Part model, mm, in its own coordinate system. Face numbers are marked on the shaded views. A direction names the side the tool comes from. Round coordinates to 2 decimals unless told otherwise and drop trailing zeros. Loops run counter-clockwise (first coordinate to the right, second up) from the corner with the lowest first, then second, coordinate; pieces in that order, holes last. Notation, with made-up numbers: (6.25, 82.25) -> (54.25, 82.25) arc R13 ccw to (54.25, 97.25) -> close; hole circle Ø1 at (-10, -27). An arc over 180 degrees is marked (long way). Answer as CSV lines item,"result".
Autodesk Inventor part; units mm, degrees
ref_plane "YZ Plane" through (0, 0, 0) normal (1, 0, 0) x (0, 1, 0)
ref_plane "XZ Plane" through (0, 0, 0) normal (0, 1, 0) x (-1, 0, 0)
ref_plane "XY Plane" through (0, 0, 0) normal (0, 0, 1) x (1, 0, 0)
sketch "Sketch1" plane through (0, 0, 0) normal (1, 0, 0) x (0, 1, 0)
  line L0 (12.954, 12.7) -> (12.954, -12.954)
  line L1 (12.954, -12.954) -> (-12.954, -12.954)
  line L2 (-12.954, -12.954) -> (-12.954, 12.7)
  line L3 (12.954, 17.78) -> (18.034, 17.78)
  line L4 (18.034, 17.78) -> (18.034, -18.034)
  line L5 (18.034, -18.034) -> (-18.034, -18.034)
  line L6 (-18.034, -18.034) -> (-18.034, 17.78)
  line L7 (-18.034, 17.78) -> (-12.954, 17.78)
  line L8 (12.954, 12.7) -> (12.954, 17.78)
  line L9 (-12.954, 12.7) -> (-12.954, 17.78)
  point P0 (0, 0)
extrude "Extrusion1" add sketch "Sketch1" along normal blind 76.2
sketch "Sketch3" plane through (76.2, 18.034, 17.78) normal (0, 1, 0) x (1, 0, 0)
  circle A0 centre (-12.7, 18.034) radius 2.4892
  line L0 (-76.2, 35.814) -> (0, 35.814)
  line L1 (0, 0) -> (0, 30.734)
  circle A1 centre (-25.4, 18.034) radius 2.4892
  circle A2 centre (-38.1, 18.034) radius 2.4892
  circle A3 centre (-50.8, 18.034) radius 2.4892
  circle A4 centre (-63.5, 18.034) radius 2.4892
  point P0 (-76.2, 17.78)
  point P1 (-63.5, 35.814)
  dimension "d11" = 4.9784
  dimension "d13" = 12.7
  dimension "d14" = 12.7
  dimension "d17" = 12.7
  dimension "d36" = 4.9784
  dimension "d37" = 12.7
extrude "Extrusion6" cut sketch "Sketch3" against normal blind 66.675
sketch "Sketch6" plane through (0, 0, 0) normal (-1, 0, 0) x (0, 0, 1)
  line L0 (-18.034, 18.034) -> (17.78, 18.034)
  line L1 (-18.034, 18.034) -> (-49.784, 18.034)
  line L2 (17.78, -18.034) -> (-18.034, -18.034)
  line L3 (-49.784, 18.034) -> (-18.034, -18.034)
  line L4 (-18.034, -18.034) -> (-18.034, 18.034)
  point P0 (0, 0)
  dimension "d40" = 31.75
extrude "Extrusion7" add sketch "Sketch6" against normal blind 25.4
sketch "Sketch7" plane through (0, 18.034, 17.78) normal (0, 1, 0) x (1, 0, 0)
  circle A0 centre (38.1, 18.034) radius 2.4892
  circle A1 centre (50.8, 18.034) radius 2.4892
  circle A2 centre (25.4, 18.034) radius 2.4892
  circle A3 centre (63.5, 18.034) radius 2.4892
  circle A4 centre (12.7, 18.034) radius 2.4892
  line L0 (0, 0) -> (0, 67.564)
  line L1 (0, 0) -> (76.2, 0)
  line L2 (76.2, 35.814) -> (76.2, 0)
  line L3 (25.4, 35.814) -> (76.2, 35.814)
  line L4 (25.4, 67.564) -> (25.4, 35.814)
  line L5 (0, 67.564) -> (25.4, 67.564)
  line L6 (0, 35.814) -> (25.4, 35.814)
  line L7 (25.4, 35.814) -> (0, 35.814)
  point P0 (0, 17.78)
extrude "Extrusion8" add sketch "Sketch7" along normal blind 88.9 contours L0 L5 L4 L6
sketch "Sketch8" plane through (25.4, 0, 0) normal (1, 0, 0) x (0, 0, -1)
  line L0 (18.034, -18.034) -> (18.034, 18.034)
  line L1 (18.034, -18.034) -> (49.784, 18.034)
  line L2 (49.784, 18.034) -> (49.784, 106.934)
  line L3 (18.034, 106.934) -> (49.784, 106.934)
  line L4 (18.034, 18.034) -> (18.034, 106.934)
  line L5 (49.784, 106.934) -> (18.034, 106.934)
  circle A0 centre (33.909, 106.934) radius 31.75
  point P0 (0, 0)
  dimension "d45" = 63.5
extrude "Extrusion9" add sketch "Sketch8" against normal up to surface (25.4 mm away) contours A0 L2 L3 L4 | L4 L3 L2 A0
sketch "Sketch9" plane through (25.4, 0, 0) normal (1, 0, 0) x (0, 0, -1)
  line L0 (18.034, 18.034) -> (18.034, 79.4377)
  line L1 (18.034, -18.034) -> (18.034, 18.034)
  line L2 (18.034, -18.034) -> (49.784, 18.034)
  line L3 (49.784, 18.034) -> (49.784, 79.4377)
  arc A0 (49.784, 79.4377) -> (18.034, 79.4377) centre (33.909, 106.934) ccw
  circle A1 centre (33.909, 106.934) radius 19.05
  circle A2 centre (33.909, 125.984) radius 3.175
  circle A3 centre (26.1607, 124.337) radius 3.175
  circle A4 centre (19.7521, 119.6809) radius 3.175
  circle A5 centre (15.7914, 112.8208) radius 3.175
  circle A6 centre (14.9634, 104.9427) radius 3.175
  circle A7 centre (17.4112, 97.409) radius 3.175
  circle A8 centre (22.7117, 91.5222) radius 3.175
  circle A9 centre (29.9483, 88.3003) radius 3.175
  circle A10 centre (37.8697, 88.3003) radius 3.175
  circle A11 centre (45.1063, 91.5222) radius 3.175
  circle A12 centre (50.4068, 97.409) radius 3.175
  circle A13 centre (52.8546, 104.9427) radius 3.175
  circle A14 centre (52.0266, 112.8208) radius 3.175
  circle A15 centre (48.0659, 119.6809) radius 3.175
  circle A16 centre (41.6573, 124.337) radius 3.175
  point P0 (0, 0)
  dimension "d48" = 38.1
  dimension "d49" = 6.35
  dimension "d52" = 360
extrude "Extrusion10" cut sketch "Sketch9" against normal blind 25.4 contours A1 A13 | A1 A13 | A14 A1 | A1 A14 | A12 A1 | A1 A12 | A15 A1 | A1 A15 | A11 A1 | A1 A11 | A16 A1 | A1 A16 | A10 A1 | A1 A10 | A2 A1 | A1 A2 | A9 A1 | A1 A9 | A3 A1 | A1 A3 | A8 A1 | A1 A8 | A4 A1 | A1 A4 | A7 A1 | A1 A7 | A5 A1 | A1 A5 | A6 A1 | A1 A6
properties part number "2024-900-004-REV2"
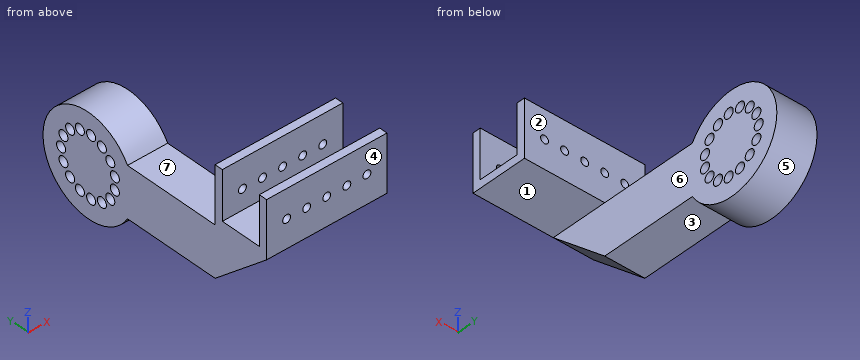
Q1. Saw through at A-A, the plane x = 50.8. Write the cut outline in (y, z), then the cut area to 3 significant figures.
Geometry results:
outline,"(-18.03, -18.03) -> (18.03, -18.03) -> (18.03, -2.74) -> (12.95, -2.74) -> (12.95, -12.95) -> (-12.95, -12.95) -> (-12.95, -2.74) -> (-18.03, -2.74) -> close; (-18.03, 2.24) -> (-12.95, 2.24) -> (-12.95, 17.78) -> (-18.03, 17.78) -> close; (12.95, 2.24) -> (18.03, 2.24) -> (18.03, 17.78) -> (12.95, 17.78) -> close"
area,"445 mm2"
Q2. Saw through at D-D, the plane z = -58.5. Write the cut outline in (x, y).
Geometry results:
outline,"(0, 86.85) -> (25.4, 86.85) -> (25.4, 127.02) -> (0, 127.02) -> close"
Q3. Saw through at B-B, the plane x = 12.7. Give the number of separate pieces and of enclosed holes in the cut face, then the cut area to 3 significant figures.
Geometry results:
separate pieces,"3"
enclosed holes,"15"
area,"5,570 mm2"
Q4. Saw through at C-C, the plane y = 36.5. Write the cut outline in (x, z), then the cut area to 3 significant figures.
Geometry results:
outline,"(0, -49.78) -> (25.4, -49.78) -> (25.4, -18.03) -> (0, -18.03) -> close"
area,"806 mm2"
Q5. Drill centre lines: line 1 along Z through (x, y) = (3.5, 121); line 2 along Z through (x, y) = (22, 93.5); line 3 along X through (y, z) = (72.5, -22). Where is each one in solid material? Low to high.
Geometry results:
line 1,"-62.37 to -50.95, -45.18 to -22.64, -16.86 to -5.44"
line 2,"-62.68 to -47.59, -42.62 to -25.2, -20.23 to -5.14"
line 3,"0 to 25.4"
Q6. Drop flat-ended pins along their axis: P1, Ø1, axis at y = 104, z = -3, coming from the +X side; P2, Ø7.5, axis at x = 17.5, y = 38.5, coming from the -Z side; P3, Ø7.5, axis at x = 14, y = 45.5, coming from the +Z side. Give the stop position or say it passes through.
Geometry results:
P1,"x = 25.4"
P2,"z = -49.78"
P3,"z = -18.03"
Q7. Which spindle directions (+Z, -Z, +X, -X, +Y, -Y) get a long thin tool onto all of the face, cutting with end or side? Do the marked faces 1, 2 and 3. Say none if no direction does.
Geometry results:
face 1,"-Z, +X, +Y, -Y"
face 2,"+Z, +X, -X"
face 3,"-Z, +X, -X, -Y"
Q8. Two-plate mould, pull along Y, no slides. Class the marked faces 4, 5, 6 and 7: pulls with the +Y half, pulls with the -Y half, needs draft (parallel to the pull), parting line crosses it, or undercut.
Geometry results:
face 4,"pulls with the -Y half"
face 5,"undercut"
face 6,"needs draft"
face 7,"undercut"
